Model file for the job. Use its own axes, mm. Face numbers are marked on the shaded views. A direction names the side the tool comes from. Coordinates: 2 decimals unless noted, no trailing zeros. Return JSON: item names as keys, results as strings.
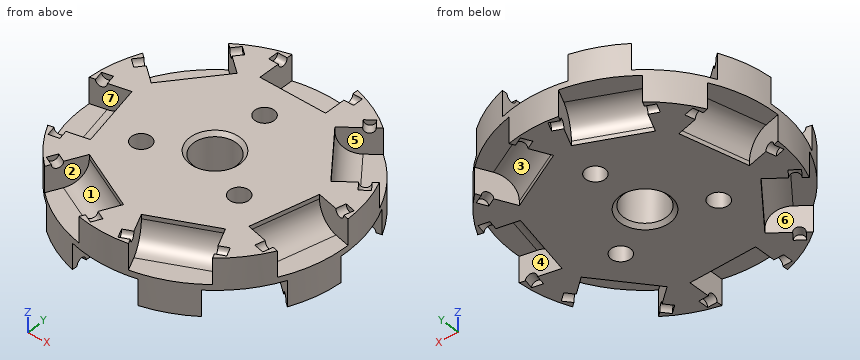
```python
from build123d import *

# Parameters (mm, degrees)
SKETCH1_R           = 29.0703
BOSS_EXTRUDE2_DEPTH = 6.35
SKETCH2_W           = 14.732
SKETCH2_H           = 10.414
CUT_EXTRUDE2_DEPTH  = 5.715
CIRPATTERN1_COUNT   = 7
SKETCH4_R           = 1.143
CUT_EXTRUDE4_DEPTH  = 9.525
CIRPATTERN2_COUNT   = 7
SKETCH5_R           = 4.7625
CUT_EXTRUDE5_DEPTH  = 42.599124801
SKETCH6_R           = 2.159
CUT_EXTRUDE7_DEPTH  = 42.599124801
BOSS_EXTRUDE3_START = 6.35
SKETCH9_R           = 29.0703
SKETCH9_R_2         = 2.159
SKETCH9_R_3         = 4.7625
BOSS_EXTRUDE3_DEPTH = 6.35
CUT_EXTRUDE8_DEPTH  = 5.715
CIRPATTERN3_COUNT   = 7
SKETCH11_R          = 1.143
CUT_EXTRUDE9_DEPTH  = 9.525
CIRPATTERN4_COUNT   = 7
FILLET1_R           = 4.7625
CHAMFER1_SIZE       = 0.79375


with BuildPart() as part:
    # Sketch1 → Boss-Extrude2 (new body)
    with BuildSketch(Plane.XY):
        Circle(SKETCH1_R)
    extrude(amount=-BOSS_EXTRUDE2_DEPTH)

    # Sketch2 → Cut-Extrude2 (cut)
    with BuildSketch(Plane.XY):
        with Locations((0, 25.1333)):
            Rectangle(SKETCH2_W, SKETCH2_H)
    cut_extrude2 = extrude(amount=-CUT_EXTRUDE2_DEPTH, mode=Mode.SUBTRACT)

    # CirPattern1: Cut-Extrude2 ×7 about axis
    cirpattern1_axis = Axis((0, 0, 0), (0, 0, 1))
    for i in range(1, CIRPATTERN1_COUNT):
        add(cut_extrude2.rotate(cirpattern1_axis, i * 360 / CIRPATTERN1_COUNT), mode=Mode.SUBTRACT)

    # Sketch4 → Cut-Extrude4 (cut, symmetric)
    with BuildSketch(Plane(origin=(0, 0, 0), x_dir=(0, 0, -1), z_dir=(1, 0, 0))):
        with Locations((0, 25.7683)):
            Circle(SKETCH4_R)
    cut_extrude4 = extrude(amount=CUT_EXTRUDE4_DEPTH, both=True, mode=Mode.SUBTRACT)

    # CirPattern2: Cut-Extrude4 ×7 about axis
    cirpattern2_axis = Axis((0, 0, 0), (0, 0, 1))
    for i in range(1, CIRPATTERN2_COUNT):
        add(cut_extrude4.rotate(cirpattern2_axis, i * 360 / CIRPATTERN2_COUNT), mode=Mode.SUBTRACT)

    # Sketch5 → Cut-Extrude5 (cut, through all)
    with BuildSketch(Plane.XY):
        Circle(SKETCH5_R)
    extrude(amount=-CUT_EXTRUDE5_DEPTH, mode=Mode.SUBTRACT)

    # Sketch6 → Cut-Extrude7 (cut, through all)
    with BuildSketch(Plane(origin=(0, 0, -6.35), x_dir=(-1, 0, 0), z_dir=(0, 0, -1))):
        with Locations((0, 12.7)):
            Circle(SKETCH6_R)
        with Locations((10.998522628, -6.35)):
            Circle(SKETCH6_R)
        with Locations((-10.998522628, -6.35)):
            Circle(SKETCH6_R)
    extrude(amount=-CUT_EXTRUDE7_DEPTH, mode=Mode.SUBTRACT)

    # Sketch9 → Boss-Extrude3 (add)
    with BuildSketch(Plane(origin=(0, 0, -6.35), x_dir=(-1, 0, 0), z_dir=(0, 0, -1)).offset(BOSS_EXTRUDE3_START)):
        with Locations(Location((0, 0, 0), (0, 0, 178.179188094))):
            Circle(SKETCH9_R)
        with Locations((0, 12.7)):
            Circle(SKETCH9_R_2, mode=Mode.SUBTRACT)
        with Locations((10.998522628, -6.35)):
            Circle(SKETCH9_R_2, mode=Mode.SUBTRACT)
        with Locations((-10.998522628, -6.35)):
            Circle(SKETCH9_R_2, mode=Mode.SUBTRACT)
        with Locations(Location((0, 0, 0), (0, 0, 180))):
            Circle(SKETCH9_R_3, mode=Mode.SUBTRACT)
    extrude(amount=-BOSS_EXTRUDE3_DEPTH)

    # Sketch10 → Cut-Extrude8 (cut)
    with BuildSketch(Plane(origin=(0, 0, -12.7), x_dir=(-1, 0, 0), z_dir=(0, 0, -1))):
        Polygon((-2.009055407, 21.148973594), (-15.282160644, 14.757064537), (-19.800579114, 24.139776859), (-6.527473878, 30.531685916), align=None)
    cut_extrude8 = extrude(amount=-CUT_EXTRUDE8_DEPTH, mode=Mode.SUBTRACT)

    # CirPattern3: Cut-Extrude8 ×7 about axis
    cirpattern3_axis = Axis((0, 0, 0), (0, 0, 1))
    for i in range(1, CIRPATTERN3_COUNT):
        add(cut_extrude8.rotate(cirpattern3_axis, i * 360 / CIRPATTERN3_COUNT), mode=Mode.SUBTRACT)

    # Sketch11 → Cut-Extrude9 (cut, symmetric)
    with BuildSketch(Plane(origin=(0, 0, 0), x_dir=(0, 0, -1), z_dir=(-0.900971031519736, 0.4338792462912495, 0))):
        with Locations((12.7, -25.7683)):
            Circle(SKETCH11_R)
    cut_extrude9 = extrude(amount=CUT_EXTRUDE9_DEPTH, both=True, mode=Mode.SUBTRACT)

    # CirPattern4: Cut-Extrude9 ×7 about axis
    cirpattern4_axis = Axis((0, 0, 0), (0, 0, 1))
    for i in range(1, CIRPATTERN4_COUNT):
        add(cut_extrude9.rotate(cirpattern4_axis, i * 360 / CIRPATTERN4_COUNT), mode=Mode.SUBTRACT)

    # Fillet1
    fillet1_edges = [part.edges().sort_by_distance(p)[0] for p in [
        (-15.579008669, 12.423844839, -5.715),
        (0, 19.9263, -5.715),
        (8.645608025, 17.953019065, -6.985),
        (-8.645787076, 17.952932839, -6.985),
        (-19.426728167, 4.433922012, -6.985),
        (-15.578946715, -12.423922526, -6.985),
        (9.9366e-05, -19.9263, -6.985),
        (15.579070622, -12.423767151, -6.985),
        (19.426683945, 4.434115761, -6.985),
        (8.645697551, -17.952975952, -5.715),
        (19.426706057, -4.434018886, -5.715),
        (-19.426706057, -4.434018886, -5.715),
        (-8.645697551, -17.952975952, -5.715),
        (15.579008669, 12.423844839, -5.715),
    ]]
    fillet(fillet1_edges, radius=FILLET1_R)

    # Chamfer1
    chamfer1_edges = [part.edges().sort_by_distance(p)[0] for p in [
        (-4.7625, 0, 0),
        (-4.7625, 0, -12.7),
    ]]
    chamfer(chamfer1_edges, length=CHAMFER1_SIZE)


solid = part.part
```
Item 1: Wall check: line 1 (Z direction, x = -21, y = -14) (3 decimals); line 2 (Z direction, x = 26.5, y = -6.5) (3 decimals); line 3 (Y direction, x = 0, z = -7.5). Give the ranges that are in metal, low to high.
Check result:
{"line 1": "z = -6.985 to 0", "line 2": "z = -12.7 to -5.715", "line 3": "y = -22.53 to -4.76, 4.76 to 10.54, 14.86 to 29.07"}
Item 2: 3-axis set-ups, long thin cutter, end or side, ignore diameter. For the marked faces 1, 2 and 3: which of +Z, -Z, +X, -X, +Y, -Y reach the whole face in a straight line?
Check result:
{"face 1": "+Z", "face 2": "+Z, -Y", "face 3": "-Z"}
Item 3: Pull direction X, two halves, no side cores. Call the marked faces 4, 5, 6 and 7: +X half, -X half, draft (parallel to the pull), parting line (faces both ways), or undercut.
Check result:
{"face 4": "undercut", "face 5": "+X half", "face 6": "-X half", "face 7": "undercut"}
Item 4: Drop flat-ended pins along their axis: pin 1 Ø6 at (y, z) = (-7, -7.5) entering from +X; pin 2 Ø1.7 at (y, z) = (-22.5, -9) entering from -X; pin 3 Ø10.5 at (x, y) = (-14.5, -24) entering from +Z; pin 4 Ø5.5 at (x, y) = (0, 0) entering from +Z. Give the stop position or say it passes through.
Check result:
{"pin 1": "stops at x = 28.79", "pin 2": "stops at x = -17.39", "pin 3": "stops at z = 0", "pin 4": "passes through"}
Item 5: Saw through at A-A (z = -8.75). Count the separate pieces of the cut face and the enclosed holes in it, and give its area (3 significant figures).
Check result:
{"separate pieces": "1", "enclosed holes": "4", "area": "1,740 mm2"}
